Design review of the part built by this model. Coordinates are the model's own, in mm. A direction names the side the tool comes from. Coordinates: 2 decimals unless noted, no trailing zeros. Loops run counter-clockwise (first coordinate to the right, second up) from the corner with the lowest first, then second, coordinate; pieces in that order, holes last. Notation, with made-up numbers: (49, 69.5) - (92, 69.5) arc R23 ccw to (92, 81.5) - close; hole circle Ø6 at (-13.5, 30.25). An arc over 180 degrees is marked (long way). One line per question, with ' | ' between items.
from build123d import *

# Parameters (mm, degrees)
BOSS_EXTRUDE1_DEPTH = 15
SKETCH18_W          = 3.3
SKETCH18_H          = 2.5
CUT_EXTRUDE10_DEPTH = 43.3
SKETCH19_W          = 3.3
SKETCH19_H          = 2.5
CUT_EXTRUDE11_DEPTH = 43.3
SKETCH20_W          = 6.221233688
SKETCH20_H          = 2.5
CUT_EXTRUDE12_DEPTH = 57.710616844
SKETCH21_W          = 6.221233688
SKETCH21_H          = 2.5
CUT_EXTRUDE13_DEPTH = 57.710616844
SKETCH22_R          = 2.5
CUT_EXTRUDE14_DEPTH = 13.5
CUT_EXTRUDE15_DEPTH = 28.5
FILLET8_R           = 6


with BuildPart() as part:
    # Sketch1 → Boss-Extrude1 (new body)
    with BuildSketch(Plane(origin=(0, 0, 0), x_dir=(1, 0, 0), z_dir=(0, 1, 0))):
        Polygon((-21.15, 16.750923472), (-16.750923472, 21.15), (16.750923472, 21.15), (21.15, 16.750923472), (21.15, -16.750923472), (16.750923472, -21.15), (-16.750923472, -21.15), (-21.15, -16.750923472), align=None)
    boss_extrude1 = extrude(amount=BOSS_EXTRUDE1_DEPTH)

    # Sketch18 → Cut-Extrude10 (cut, through all)
    with BuildSketch(Plane.XY.offset(21.15)):
        with Locations((15.100923472, 13.75)):
            Rectangle(SKETCH18_W, SKETCH18_H)
        with Locations((-15.100923472, 13.75)):
            Rectangle(SKETCH18_W, SKETCH18_H)
    cut_extrude10 = extrude(amount=-CUT_EXTRUDE10_DEPTH, mode=Mode.SUBTRACT)

    # Sketch19 → Cut-Extrude11 (cut, through all)
    with BuildSketch(Plane(origin=(21.15, 0, 0), x_dir=(0, 0, -1), z_dir=(1, 0, 0))):
        with Locations((-15.100923472, 13.75)):
            Rectangle(SKETCH19_W, SKETCH19_H)
        with Locations((15.100923472, 13.75)):
            Rectangle(SKETCH19_W, SKETCH19_H)
    cut_extrude11 = extrude(amount=-CUT_EXTRUDE11_DEPTH, mode=Mode.SUBTRACT)

    # Sketch20 → Cut-Extrude12 (cut, through all)
    with BuildSketch(Plane(origin=(18.950461736, 0, 18.950461736), x_dir=(0.707106781, 0, -0.707106781), z_dir=(0.707106781, 0, 0.707106781))):
        with Locations((0, 13.75)):
            Rectangle(SKETCH20_W, SKETCH20_H)
    cut_extrude12 = extrude(amount=-CUT_EXTRUDE12_DEPTH, mode=Mode.SUBTRACT)

    # Sketch21 → Cut-Extrude13 (cut, through all)
    with BuildSketch(Plane(origin=(-18.950461736, 0, 18.950461736), x_dir=(0.707106781, 0, 0.707106781), z_dir=(-0.707106781, 0, 0.707106781))):
        with Locations((0, 13.75)):
            Rectangle(SKETCH21_W, SKETCH21_H)
    cut_extrude13 = extrude(amount=-CUT_EXTRUDE13_DEPTH, mode=Mode.SUBTRACT)

    # Sketch22 → Cut-Extrude14 (cut, through all)
    with BuildSketch(Plane(origin=(0, 12.5, 0), x_dir=(1, 0, 0), z_dir=(0, 1, 0))):
        Circle(SKETCH22_R)
    cut_extrude14 = extrude(amount=-CUT_EXTRUDE14_DEPTH, mode=Mode.SUBTRACT)

    # Mirror1: Boss-Extrude1, Cut-Extrude10, Cut-Extrude11, Cut-Extrude12, Cut-Extrude13, Cut-Extrude14 across plane
    add(boss_extrude1.mirror(Plane(origin=(0, 0, 0), x_dir=(0, 0, 1), z_dir=(0, -1, 0))))
    add(cut_extrude10.mirror(Plane(origin=(0, 0, 0), x_dir=(0, 0, 1), z_dir=(0, -1, 0))), mode=Mode.SUBTRACT)
    add(cut_extrude11.mirror(Plane(origin=(0, 0, 0), x_dir=(0, 0, 1), z_dir=(0, -1, 0))), mode=Mode.SUBTRACT)
    add(cut_extrude12.mirror(Plane(origin=(0, 0, 0), x_dir=(0, 0, 1), z_dir=(0, -1, 0))), mode=Mode.SUBTRACT)
    add(cut_extrude13.mirror(Plane(origin=(0, 0, 0), x_dir=(0, 0, 1), z_dir=(0, -1, 0))), mode=Mode.SUBTRACT)
    add(cut_extrude14.mirror(Plane(origin=(0, 0, 0), x_dir=(0, 0, 1), z_dir=(0, -1, 0))), mode=Mode.SUBTRACT)

    # Sketch23 → Cut-Extrude15 (cut, through all)
    with BuildSketch(Plane(origin=(0, 12.5, 0), x_dir=(1, 0, 0), z_dir=(0, 1, 0))):
        Polygon((-21.15, -14.432485579), (-14.432485579, -21.15), (-16.750923472, -21.15), (-21.15, -16.750923472), align=None)
        Polygon((-21.15, 14.432485579), (-14.432485579, 21.15), (-16.750923472, 21.15), (-21.15, 16.750923472), align=None)
        Polygon((14.432485579, 21.15), (21.15, 14.432485579), (21.15, 16.750923472), (16.750923472, 21.15), align=None)
        Polygon((14.432485579, -21.15), (21.15, -14.432485579), (21.15, -16.750923472), (16.750923472, -21.15), align=None)
    extrude(amount=-CUT_EXTRUDE15_DEPTH, mode=Mode.SUBTRACT)

    # Fillet8
    fillet8_edges = [part.edges().sort_by_distance(p)[0] for p in [
        (14.432485579, 0, -21.15),
        (21.15, 0, -14.432485579),
        (-21.15, 0, -14.432485579),
        (-14.432485579, 0, -21.15),
        (-14.432485579, 0, 21.15),
        (-21.15, 0, 14.432485579),
        (21.15, 0, 14.432485579),
        (14.432485579, 0, 21.15),
    ]]
    fillet(fillet8_edges, radius=FILLET8_R)


solid = part.part
Q1. Tool access review of faces 1 (the flat face through (19, -14, -13.451)), 2 (the flat face through (12.9, -13.7, -17.3)), 3 (the flat face through (8.9, 13.7, -4.5)), 4 (the flat face through (-13.451, 14, -19)), 5 (the flat face through (-16.751, -14, 0)): name each direction out of +Z, -Z, +X, -X, +Y, -Y from which nothing blocks a thin tool from reaching the whole face with its end or side.
Returned:
face 1: -Z, +X, -X, -Y | face 2: +X, -Y | face 3: +Y | face 4: +Z, -Z, -X, +Y | face 5: +Z, -Z, -Y
Q2. For pin 1 (10 mm diameter, centred on y = 6, z = 13, fed in from +X); pin 2 (1.2 mm diameter, centred on x = 19, y = -14, fed in from -Z); pin 3 (3 mm diameter, centred on y = -13.5, z = 19.5, fed in from -X); pin 4 (3 mm diameter, centred on y = -14.5, z = 19.5, fed in from +X), all flat-tipped, find the tip position at first contact; note any pin that passes through.
Returned:
pin 1: stops at x = 21.15 | pin 2: stops at z = -13.45 | pin 3: stops at x = -17.2 | pin 4: stops at x = 13.45
Q3. Take a section at A-A (x = 10). Give the boundary of the cut face in (y, z).
Returned:
outline: (-15, -21.15) - (15, -21.15) - (15, -16.75) - (12.5, -16.75) - (12.5, -5.6) - (15, -5.6) - (15, 5.6) - (12.5, 5.6) - (12.5, 16.75) - (15, 16.75) - (15, 21.15) - (-15, 21.15) - (-15, 16.75) - (-12.5, 16.75) - (-12.5, 5.6) - (-15, 5.6) - (-15, -5.6) - (-12.5, -5.6) - (-12.5, -16.75) - (-15, -16.75) - close
Q4. Take a section at C-C (x = 3.5). Give the boundary of the cut face in (y, z), plus the area to 3 significant figures.
Returned:
outline: (-15, -21.15) - (15, -21.15) - (15, -16.75) - (12.5, -16.75) - (12.5, -13.45) - (15, -13.45) - (15, -7.9) - (12.5, -7.9) - (12.5, 7.9) - (15, 7.9) - (15, 13.45) - (12.5, 13.45) - (12.5, 16.75) - (15, 16.75) - (15, 21.15) - (-15, 21.15) - (-15, 16.75) - (-12.5, 16.75) - (-12.5, 13.45) - (-15, 13.45) - (-15, 7.9) - (-12.5, 7.9) - (-12.5, -7.9) - (-15, -7.9) - (-15, -13.45) - (-12.5, -13.45) - (-12.5, -16.75) - (-15, -16.75) - close | area: 1,160 mm²
Q5. Take a section at B-B (z = -11). Give the boundary of the cut face in (x, y).
Returned:
outline: (-21.15, -15) - (-16.75, -15) - (-16.75, -12.5) - (-6.6, -12.5) - (-6.6, -15) - (6.6, -15) - (6.6, -12.5) - (16.75, -12.5) - (16.75, -15) - (21.15, -15) - (21.15, 15) - (16.75, 15) - (16.75, 12.5) - (6.6, 12.5) - (6.6, 15) - (-6.6, 15) - (-6.6, 12.5) - (-16.75, 12.5) - (-16.75, 15) - (-21.15, 15) - close
Q6. To check wall thickness, follow line 1 along X through (y, z) = (-10, 0); line 2 along Y through (x, z) = (-11.5, -16.5). State the ranges of each line that lie inside material, in increasing order.
Returned:
line 1: x = -21.15 to -2.5, 2.5 to 21.15 | line 2: y = -12.5 to 12.5
Q7. Draft analysis for pull direction Z (two halves, no side actions). For faces 6 (the flat face through (12.9, -13.7, 17.3)), 7 (the flat face through (-19, -14, -13.451)), 8 (the flat face through (-13.451, -14, 19)), 9 (the flat face through (9, 13.7, 4.6)), state which applies: +Z half, -Z half, draft (parallel to the pull), parting line (faces both ways), or undercut.
Returned:
face 6: undercut | face 7: -Z half | face 8: draft | face 9: undercut
